The model under review builds one solid part; all positions refer to its coordinate system, in mm. Face numbers are marked on the shaded views. A direction names the side the tool comes from. Round coordinates to 2 decimals unless told otherwise and drop trailing zeros. Loops run counter-clockwise (first coordinate to the right, second up) from the corner with the lowest first, then second, coordinate; pieces in that order, holes last. Notation, with made-up numbers: (79.5, 0) - (134.5, 0) arc R20 cw to (134.5, 25) - close; hole circle Ø11 at (18.25, -1). An arc over 180 degrees is marked (long way). Answer as CSV lines item,"result".
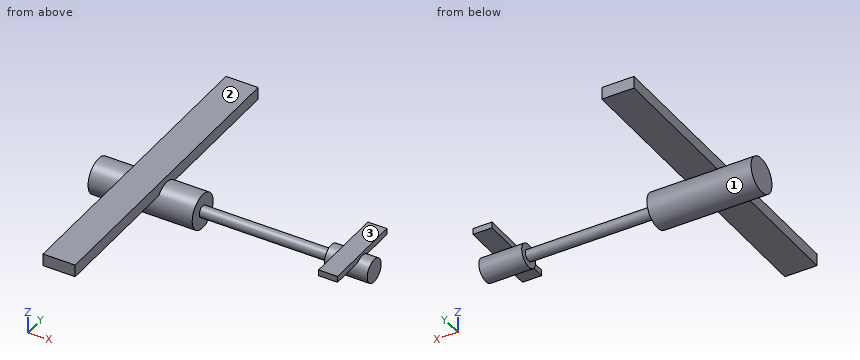
from build123d import *

# Parameters (mm, degrees)
SKETCH2_R           = 57.15
BOSS_EXTRUDE1_DEPTH = 340
SKETCH3_R           = 18.53927994
BOSS_EXTRUDE2_DEPTH = 420
SKETCH4_R           = 38.1
BOSS_EXTRUDE3_DEPTH = 140
SKETCH5_W           = 105
SKETCH5_H           = 40
BOSS_EXTRUDE4_DEPTH = 500
SKETCH6_W           = 62.2
SKETCH6_H           = 20
BOSS_EXTRUDE5_DEPTH = 135


with BuildPart() as part:
    # Sketch2 → Boss-Extrude1 (new body)
    with BuildSketch(Plane.YZ):
        with Locations(Location((0, 0, 0), (0, 0, 270))):
            Circle(SKETCH2_R)
    extrude(amount=BOSS_EXTRUDE1_DEPTH)

    # Sketch3 → Boss-Extrude2 (add)
    with BuildSketch(Plane.YZ.offset(340)):
        with Locations(Location((0, 0, 0), (0, 0, 270))):
            Circle(SKETCH3_R)
    extrude(amount=BOSS_EXTRUDE2_DEPTH)

    # Sketch4 → Boss-Extrude3 (add)
    with BuildSketch(Plane.YZ.offset(760)):
        with Locations(Location((0, 0, 0), (0, 0, 270))):
            Circle(SKETCH4_R)
    extrude(amount=BOSS_EXTRUDE3_DEPTH)

    # Sketch5 → Boss-Extrude4 (add, symmetric)
    with BuildSketch(Plane(origin=(0, 0, 0), x_dir=(-1, 0, 0), z_dir=(0, 1, 0))):
        with Locations((-170, 57.15)):
            Rectangle(SKETCH5_W, SKETCH5_H)
    extrude(amount=BOSS_EXTRUDE4_DEPTH, both=True)

    # Sketch6 → Boss-Extrude5 (add, symmetric)
    with BuildSketch(Plane(origin=(0, 0, 0), x_dir=(-1, 0, 0), z_dir=(0, 1, 0))):
        with Locations((-830, 38.1)):
            Rectangle(SKETCH6_W, SKETCH6_H)
    extrude(amount=BOSS_EXTRUDE5_DEPTH, both=True)


solid = part.part
1. Take a section at D-D (y = -193). State the section outline as (x, z) points.
Numbers:
outline,"(117.5, 37.15) - (222.5, 37.15) - (222.5, 77.15) - (117.5, 77.15) - close"
2. Clearance check with flat-ended pins moving along their axes: pin 1 (6 mm diameter, centred on y = 30.5, z = 34, fed in from +X); pin 2 (12 mm diameter, centred on y = 188, z = 57, fed in from +X); pin 3 (4 mm diameter, centred on x = 810, z = 29.5, fed in from -Y); pin 4 (10 mm diameter, centred on y = 43.5, z = 39, fed in from -X). State where each tip first meets the part, or that it passes through.
Numbers:
pin 1,"stops at x = 861.1"
pin 2,"stops at x = 222.5"
pin 3,"stops at y = -135"
pin 4,"stops at x = 0"
3. Take a section at A-A (y = 0). State the section outline as (x, z) points, plus the area to 3 significant figures.
Numbers:
outline,"(0, -57.15) - (340, -57.15) - (340, -18.54) - (760, -18.54) - (760, -38.1) - (900, -38.1) - (900, 38.1) - (861.1, 38.1) - (861.1, 48.1) - (798.9, 48.1) - (798.9, 38.1) - (760, 38.1) - (760, 18.54) - (340, 18.54) - (340, 57.15) - (222.5, 57.15) - (222.5, 77.15) - (117.5, 77.15) - (117.5, 57.15) - (0, 57.15) - close"
area,"67,800 mm²"
4. Take a section at B-B (z = 0). State the section outline as (x, y) points, plus the area to 3 significant figures.
Numbers:
outline,"(0, -57.15) - (340, -57.15) - (340, -18.54) - (760, -18.54) - (760, -38.1) - (900, -38.1) - (900, 38.1) - (760, 38.1) - (760, 18.54) - (340, 18.54) - (340, 57.15) - (0, 57.15) - close"
area,"65,100 mm²"
5. Take a section at C-C (x = 562.5). State the section outline as (y, z) points, plus the area to 3 significant figures.
Numbers:
outline,"circle Ø37.08 at (0, 0)"
area,"1,080 mm²"
6. Wall thickness on probe 1 along X at (y, z) = (-29, 20); probe 2 along X at (y, z) = (-34.5, 39.5); probe 3 along X at (y, z) = (-410.5, 55): over which ranges is each line inside the solid? List them lowest first.
Numbers:
probe 1,"x = 0 to 340, 760 to 900"
probe 2,"x = 0 to 340, 798.9 to 861.1"
probe 3,"x = 117.5 to 222.5"
7. Tool access review of the marked faces 1, 2 and 3: name each direction out of +Z, -Z, +X, -X, +Y, -Y from which nothing blocks a thin tool from reaching the whole face with its end or side.
Numbers:
face 1,"none"
face 2,"+Z, +X, -X, +Y, -Y"
face 3,"+Z, +X, +Y, -Y"
